The listing builds one solid part. Answer for the finished solid, in the listing's coordinates (mm). Coordinates: 2 decimals unless noted, no trailing zeros. Loops run counter-clockwise (first coordinate to the right, second up) from the corner with the lowest first, then second, coordinate; pieces in that order, holes last. Notation, with made-up numbers: (46.5, 84) - (102.5, 84) arc R17 ccw to (102.5, 91) - close; hole circle Ø10 at (1.5, -3.75). An arc over 180 degrees is marked (long way). Return JSON: item names as keys, results as strings. Group by question number.
1. The mould has two halves that part along X. Classify faces 1 (the face through (32.66, 0.78, 24.49)), 2 (the face through (-32.66, 0.78, -24.49)), 3 (the face through (-1, 1.588, -1)): pulls with the +X half, pulls with the -X half, needs draft (parallel to the pull), parting line crosses it, or undercut.
2. Section A-A (z = -25.4) is taken. Write down the section's boundary in (x, y), and give its area (3 significant figures).
3. Section C-C (z = -11) is taken. Write down the section's boundary in (x, y), and give its area (3 significant figures).
4. Section B-B (y = 1.25) is taken. Write down the section's boundary in (x, z).
5. Find the intervals of material crossed by line 1 along X through (y, z) = (0.45, -25.4); line 2 along Z through (x, y) = (33.85, 0.85); line 3 along X through (y, z) = (0.2, 26), in increasing order.
6. Each of these flat-tipped pins is pushed along its axis until it touches: P1, Ø12, axis at x = -1.5, z = 28.5, coming from the -Y side; P2, Ø0.8, axis at y = 1, z = 0, coming from the -X side; P3, Ø0.8, axis at y = 1, z = -39, coming from the +X side. Where does it stop, or does it pass through?
```python
from build123d import *

# Parameters (mm, degrees)
SKETCH1_R               = 1.5
BOSS_EXTRUDE1_DEPTH     = 1.5875
MIRROR2_COPY_1_SKETCH_R = 1.5
MIRROR2_COPY_1_DEPTH    = 1.5875


with BuildPart() as part:
    # Sketch1 → Boss-Extrude1 (new body)
    with BuildSketch(Plane(origin=(0, 0, 0), x_dir=(1, 0, 0), z_dir=(0, 1, 0))):
        with BuildLine():
            Line((-27.5, -42.5), (27.5, -42.5))
            Line((27.5, -42.5), (27.5, 12.7))
            ThreePointArc((27.5, 12.7), (29.359871939, 17.190128061), (33.85, 19.05))
            ThreePointArc((33.85, 19.05), (40.2, 25.4), (33.85, 31.75))
            ThreePointArc((33.85, 31.75), (29.359871939, 33.609871939), (27.5, 38.1))
            Line((27.5, 38.1), (27.5, 42.5))
            Line((27.5, 42.5), (-27.5, 42.5))
            Line((-27.5, 42.5), (-27.5, -42.5))
        make_face()
        with Locations((33.85, 25.4)):
            Circle(SKETCH1_R, mode=Mode.SUBTRACT)
    boss_extrude1 = extrude(amount=BOSS_EXTRUDE1_DEPTH)

    # Mirror1: Boss-Extrude1 across plane
    add(boss_extrude1.mirror(Plane.XY))

    # Mirror2: Boss-Extrude1 across plane
    add(boss_extrude1.mirror(Plane(origin=(0, 0, 0), x_dir=(0, 0, 1), z_dir=(1, 0, 0))))

    # Mirror2 copy 1 sketch → Mirror2 copy 1 (add)
    with BuildSketch(Plane(origin=(0, 0, 0), x_dir=(-1, 0, 0), z_dir=(0, 1, 0))):
        with BuildLine():
            Line((-27.5, -42.5), (27.5, -42.5))
            Line((27.5, -42.5), (27.5, 12.7))
            ThreePointArc((27.5, 12.7), (29.359871939, 17.190128061), (33.85, 19.05))
            ThreePointArc((33.85, 19.05), (40.2, 25.4), (33.85, 31.75))
            ThreePointArc((33.85, 31.75), (29.359871939, 33.609871939), (27.5, 38.1))
            Line((27.5, 38.1), (27.5, 42.5))
            Line((27.5, 42.5), (-27.5, 42.5))
            Line((-27.5, 42.5), (-27.5, -42.5))
        make_face()
        with Locations((33.85, 25.4)):
            Circle(MIRROR2_COPY_1_SKETCH_R, mode=Mode.SUBTRACT)
    extrude(amount=MIRROR2_COPY_1_DEPTH)


solid = part.part
```
The answers:
{
 "1": {"face 1": "undercut", "face 2": "undercut", "face 3": "needs draft"},
 "2": {"outline": "(-40.2, 0) - (-35.35, 0) - (-35.35, 1.59) - (-40.2, 1.59) - close; (-32.35, 0) - (32.35, 0) - (32.35, 1.59) - (-32.35, 1.59) - close; (35.35, 0) - (40.2, 0) - (40.2, 1.59) - (35.35, 1.59) - close", "area": "118 mm2"},
 "3": {"outline": "(-27.5, 0) - (27.5, 0) - (27.5, 1.59) - (-27.5, 1.59) - close", "area": "87.3 mm2"},
 "4": {"outline": "(-33.85, -31.75) arc R6.35 cw to (-27.5, -38.1) - (-27.5, -42.5) - (27.5, -42.5) - (27.5, -38.1) arc R6.35 cw to (33.85, -31.75) arc R6.35 ccw to (33.85, -19.05) arc R6.35 cw to (27.5, -12.7) - (27.5, 12.7) arc R6.35 cw to (33.85, 19.05) arc R6.35 ccw to (33.85, 31.75) arc R6.35 cw to (27.5, 38.1) - (27.5, 42.5) - (-27.5, 42.5) - (-27.5, 38.1) arc R6.35 cw to (-33.85, 31.75) arc R6.35 ccw to (-33.85, 19.05) arc R6.35 cw to (-27.5, 12.7) - (-27.5, -12.7) arc R6.35 cw to (-33.85, -19.05) arc R6.35 ccw to start; hole circle Ø3 at (-33.85, -25.4); hole circle Ø3 at (-33.85, 25.4); hole circle Ø3 at (33.85, -25.4); hole circle Ø3 at (33.85, 25.4)"},
 "5": {"line 1": "x = -40.2 to -35.35, -32.35 to 32.35, 35.35 to 40.2", "line 2": "z = -31.75 to -26.9, -23.9 to -19.05, 19.05 to 23.9, 26.9 to 31.75", "line 3": "x = -40.17 to -35.22, -32.48 to 32.48, 35.22 to 40.17"},
 "6": {"P1": "stops at y = 0", "P2": "stops at x = -27.5", "P3": "stops at x = 27.5"}
}
